Autodesk Inventor part; units mm, degrees
ref_plane "YZ Plane" through (0, 0, 0) normal (1, 0, 0) x (0, 1, 0)
ref_plane "XZ Plane" through (0, 0, 0) normal (0, 1, 0) x (-1, 0, 0)
ref_plane "XY Plane" through (0, 0, 0) normal (0, 0, 1) x (1, 0, 0)
sketch "Sketch1" plane through (0, 0, 0) normal (0, 0, 1) x (1, 0, 0)
  line L0 (177.0985, -0.0099) -> (177.0985, 299.9901)
  line L1 (177.0985, 299.9901) -> (-0.7015, 299.9901) construction
  line L2 (-0.7015, 299.9901) -> (-0.7015, 12.8831)
  line L3 (3.1985, 12.8831) -> (5.7502, 12.8831)
  arc A0 (162.2875, 38.1203) -> (54.7536, 57.5761) centre (107.4018, 41.6649) ccw
  arc A1 (11.9285, 13.8613) -> (54.7536, 57.5761) centre (-8.4768, 76.6855) ccw
  arc A2 (5.7502, 12.8831) -> (11.9285, 13.8613) centre (5.7502, 32.8831) ccw
  circle A3 centre (164.4485, 93.4388) radius 2.8
  circle A4 centre (164.4485, 176.4531) radius 2.8
  circle A5 centre (164.4485, 259.4675) radius 2.8
  circle A6 centre (11.9485, 259.4675) radius 2.8
  circle A7 centre (11.9485, 176.4531) radius 2.8
  circle A8 centre (11.9485, 93.4388) radius 2.8
  arc A9 (162.2875, 38.1203) -> (169.4999, 9.3715) centre (210.7223, 34.9923) ccw
  line L4 (83.4018, 393.7) -> (83.4018, -22.225) construction
  line L5 (83.4018, -22.225) -> (131.4018, -22.225) construction
  line L6 (131.4018, -22.225) -> (131.4018, 393.7) construction
  line L7 (131.4018, 393.7) -> (83.4018, 393.7) construction
  line L8 (83.4018, 393.7) -> (131.4018, -22.225) construction
  line L9 (83.4018, -22.225) -> (131.4018, 393.7) construction
  line L10 (36.4143, 133.6649) -> (149.1268, 133.6649) construction
  line L11 (41.1768, 101.6649) -> (144.3643, 101.6649) construction
  circle A10 centre (63.4018, 133.6649) radius 1.75
  circle A11 centre (63.4018, 101.6649) radius 1.75
  line L12 (63.4018, 133.6649) -> (63.4018, 101.6649) construction
  line L13 (107.4018, 31.6649) -> (107.4018, 185.7375) construction
  circle A12 centre (107.4018, 133.6649) radius 1.75
  circle A13 centre (107.4018, 101.6649) radius 1.75
  circle A14 centre (151.4018, 133.6649) radius 1.75
  circle A15 centre (151.4018, 101.6649) radius 1.75
  line L14 (151.4018, 133.6649) -> (151.4018, 101.6649) construction
  line L15 (173.1985, 301.3071) -> (173.1985, 10.4273)
  line L16 (177.0985, -0.0099) -> (177.0985, 42.269)
  line L17 (3.1985, 301.3071) -> (3.1985, 12.8831)
  line L18 (-0.7015, 12.8831) -> (-0.7015, 42.269)
  line L19 (24.0985, 301.3071) -> (-0.2015, 301.3071)
  line L20 (3.1985, 301.3071) -> (173.1985, 301.3071)
  line L21 (177.0985, 301.3071) -> (177.0985, 299.9901)
  line L22 (177.0985, 299.9901) -> (-0.7015, 299.9901) construction
  line L23 (-0.7015, 299.9901) -> (-0.7015, 301.3071)
  circle A16 centre (107.4018, 41.6649) radius 50.5415
  circle A17 centre (137.6518, 94.0594) radius 2.8
  line L24 (137.6518, 94.0594) -> (107.4018, 41.6649) construction
  line L25 (107.4018, 41.6649) -> (75.7506, 96.4865) construction
  circle A18 centre (77.1518, 94.0594) radius 2.8
  arc A19 (169.4999, 9.3715) -> (173.1985, 10.4273) centre (171.1985, 10.4273) ccw
  circle A20 centre (100.0728, 157.9036) radius 4.75
  circle A21 centre (68.0733, 158.0877) radius 4.75
  circle A22 centre (100.0728, 157.9036) radius 2.8
  circle A23 centre (68.0733, 158.0877) radius 2.8
  point P0 (0, 0)
  point P1 (152.4018, -0.0099)
  point P2 (173.1985, 42.269)
  point P3 (3.1985, 42.269)
  point P4 (174.0985, 3.1425)
  point P5 (24.0985, 301.3071)
  point P6 (173.1985, 4.2079)
  dimension "d0" = 177.8
  dimension "d1" = 300
  dimension "d9" = 258.3252
  dimension "d10" = 55
  dimension "d11" = 108.1033
  dimension "d12" = 48
  dimension "d13" = 32
  dimension "d14" = 3.5
  dimension "d15" = 3.5
  dimension "d16" = 20
  dimension "d17" = 3.5
  dimension "d18" = 3.5
  dimension "d19" = 3.5
  dimension "d20" = 3.5
  dimension "d21" = 20
  dimension "d22" = 3.9
  dimension "d23" = 3.9
  dimension "d24" = 60
  dimension "d25" = 5.6
  dimension "d26" = 60.5
  dimension "d27" = 60
  dimension "d28" = 60
  dimension "d29" = 5.6
  dimension "d30" = 60.5
  dimension "d31" = 2
  dimension "d32" = 5.6
  dimension "d33" = 5.6
extrude "Extrusion1" add sketch "Sketch1" along normal blind 6.35 contours L17 L19 L20 L15 A19 A9 A0 A1 A2 L3 | A20 | A21
equation "\"d21\" = d16"
equation "\"d30\" = d26"
properties part number "Lower Deck" material "Polycarbonate, Clear"
Input: part model. Units: mm. Frame: model coordinates. A direction names the side the tool comes from. Give positions to 0.01 mm unless a question says otherwise; leave off trailing zeros. Order: outer loops, then holes, each group sorted by start corner. A loop starts at its lowest first (then second) coordinate and runs counter-clockwise, first axis right, second up. Notation, with made-up numbers: M 1,10.25 L 42,10.25 A31 ccw 42,34.25 Z; hole C 1,-39.75 d1. An arc over 180 degrees is marked long. One line per question, with ' | ' between items. Start each with the question number.
1. First-contact query: pin 1 Ø4.5 at (x, y) = (151.4, 133.66) entering from +Z. Flat tip, straight axial feed; report the tip coordinate or a pass-through.
2. Section query B-B (x = 20.5). Return the cut outline in (y, z), and give its area (3 significant figures).
3. Pull-direction query (Y, two-part tool) for faces 3 (the face through (11.584, 90.663, 3.131)), 4 (the face through (8.921, 13.136, 3.131)), 5 (the face through (3.198, 159, 3)), 6 (the face through (89, 301.307, 3)); classes: released by +Y, released by -Y, zero draft, split by the parting line, or undercut.
4. Section query A-A (z = 3.5). Count the separate pieces of the cut face and the enclosed holes in it, and give its area (3 significant figures).
5. Section query C-C (x = 84). Return the cut outline in (y, z).
6. Access query for faces 1 (the face through (87, 189, 6.35)), 2 (the face through (39.02, 30.78, 3.13)). Directions: +Z, -Z, +X, -X, +Y, -Y. A direction counts if a zero-diameter tool reaches every point of the face in a straight line with its end or side. Return the directions, or none.
7. Material intervals for probe 1 along X at (y, z) = (257.5, 3); probe 2 along X at (y, z) = (62, 2.75); probe 3 along Y at (x, z) = (98.5, 2.5), sorted ascending. Write a range as [from, to].
Here are the results:
1) pin 1: z = 6.35
2) outline: M 17.33,0 L 301.31,0 L 301.31,6.35 L 17.33,6.35 Z | area: 1,800 mm²
3) face 3: undercut | face 4: released by -Y | face 5: zero draft | face 6: released by +Y
4) separate pieces: 1 | enclosed holes: 16 | area: 40,200 mm²
5) outline: M 91.44,0 L 301.31,0 L 301.31,6.35 L 91.44,6.35 Z
6) face 1: +Z, +X, -X, +Y, -Y | face 2: +Z, -Z, -Y
7) probe 1: [3.2, 9.96], [13.94, 162.46], [166.44, 173.2] | probe 2: [3.2, 56.3], [158.5, 173.2] | probe 3: [95.94, 155.59], [160.22, 301.31]
